from build123d import *


with BuildPart() as part:
    # Эскиз1 → Повернуть1 (revolve)
    with BuildSketch(Plane(origin=(0, 0, 0), x_dir=(0, 0, -1), z_dir=(1, 0, 0))):
        Polygon((0, 0), (0, -40.5), (4, -40.5), (4, -31.5), (10, -31.5), (10, 0), align=None)
    revolve_1 = revolve(axis=Axis((0, -1000, 0), (0, 1, 0)))

    # Зеркальное отражение1: Повернуть1 across plane
    add(revolve_1.mirror(Plane(origin=(0, 0, -10), x_dir=(0, 0, 1), z_dir=(0, 1, 0))))


solid = part.part
Part model, mm, in its own coordinate system. A direction names the side the tool comes from. Coordinates: 2 decimals unless noted, no trailing zeros. Write each loop counter-clockwise with the first axis right and the second up, starting at its lowest first coordinate (ties: lowest second). Pieces come first, ordered by that corner, then holes. Notation, with made-up numbers: (-33, 4) - (19, 4) arc R31 ccw to (19, 38) - close; hole circle Ø10 at (88.5, 26). An arc over 180 degrees is marked (long way). Put each result on its own line as item: value.
1. 3-axis set-ups, long thin cutter, end or side, ignore diameter. For faces 1 (the flat face through (0, 40.5, 0)), 2 (the cylindrical face through (3.905, 35.937, 0.867)), 3 (the cylindrical face through (3.905, -35.937, 0.867)): which of +Z, -Z, +X, -X, +Y, -Y reach the whole face in a straight line?
Final values:
face 1: +Z, -Z, +X, -X, +Y
face 2: +Y
face 3: -Y
2. Probe line 1 along Y through (x, z) = (0.25, -8); line 2 along Z through (x, y) = (0.25, 0); line 3 along Z through (x, y) = (-6, 26.5). List the from-to ranges inside material, lowest first. Write a range as [from, to].
Final values:
line 1: y = [-31.5, 31.5]
line 2: z = [-10, 10]
line 3: z = [-8, 8]
3. Band-saw the part on B-B (x = 0). Write the cut outline in (y, z).
Final values:
outline: (-40.5, -4) - (-31.5, -4) - (-31.5, -10) - (31.5, -10) - (31.5, -4) - (40.5, -4) - (40.5, 4) - (31.5, 4) - (31.5, 10) - (-31.5, 10) - (-31.5, 4) - (-40.5, 4) - close
4. Flat gauge pins, fed straight in: pin 1 Ø2 at (y, z) = (21, 7) entering from -X; pin 2 Ø1.5 at (x, y) = (1.5, 6.5) entering from +Z; pin 3 Ø5 at (y, z) = (15, 6) entering from -X. Where does each tip first touch, or does it go through?
Final values:
pin 1: stops at x = -8
pin 2: stops at z = 9.97
pin 3: stops at x = -9.37
5. Band-saw the part on D-D (z = -6). Write the cut outline in (x, y).
Final values:
outline: (-8, -31.5) - (8, -31.5) - (8, 31.5) - (-8, 31.5) - close
6. Band-saw the part on A-A (z = 0). Write the cut outline in (x, y).
Final values:
outline: (-10, -31.5) - (-4, -31.5) - (-4, -40.5) - (4, -40.5) - (4, -31.5) - (10, -31.5) - (10, 31.5) - (4, 31.5) - (4, 40.5) - (-4, 40.5) - (-4, 31.5) - (-10, 31.5) - close
7. Band-saw the part on C-C (y = -12). Write the cut outline in (x, z), then the cut area to 3 significant figures.
Final values:
outline: circle Ø20 at (0, 0)
area: 314 mm²
